Build history of the part. All positions in model axes, mm. A direction names the side the tool comes from. Round coordinates to 2 decimals unless told otherwise and drop trailing zeros. Write each loop counter-clockwise with the first axis right and the second up, starting at its lowest first coordinate (ties: lowest second). Pieces come first, ordered by that corner, then holes. Notation, with made-up numbers: (55, 9) -> (98, 9) arc R31 cw to (98, 44) -> close; hole circle Ø1 at (5, 22.25). An arc over 180 degrees is marked (long way). One line per question, with ' | ' between items.
from build123d import *

# Parameters (mm, degrees)
F0_W     = 63.5
F0_H     = 38.1
F1_DEPTH = 25.4
F3_DEPTH = 25.4


with BuildPart() as f1:
    # F0 (on Front) → F1 (new body)
    with BuildSketch(Plane.XZ):
        with Locations((-31.75, 19.05)):
            Rectangle(F0_W, F0_H)
    extrude(amount=F1_DEPTH)

    # F2 (on face) → F3 (cut)
    with BuildSketch(Plane.XZ.offset(25.4)):
        with BuildLine():
            ThreePointArc((-50.8, 38.1), (-44.931719, 24.918281), (-31.75, 19.05))
            ThreePointArc((-31.75, 19.05), (-18.530061, 24.880061), (-12.7, 38.1))
            Line((-12.7, 38.1), (-31.75, 38.1))
            Line((-31.75, 38.1), (-50.8, 38.1))
        make_face()
    extrude(amount=-F3_DEPTH, mode=Mode.SUBTRACT)


solid = f1.part
(1) 3-axis set-ups, long thin cutter, end or side, ignore diameter. For faces 1 (the cylindrical face through (-45.08, -12.88, 25.07)), 2 (the flat face through (-32, -13, 0)): which of +Z, -Z, +X, -X, +Y, -Y reach the whole face in a straight line?
Calculated:
face 1: +Z, +Y, -Y | face 2: -Z, +X, -X, +Y, -Y
(2) Slice it at C-C (x = -46.5). Write the cut outline in (y, z).
Calculated:
outline: (-25.4, 0) -> (0, 0) -> (0, 26.68) -> (-25.4, 26.68) -> close
(3) Slice it at D-D (z = 33). Write the cut outline in (x, y).
Calculated:
outline: (-63.5, -25.4) -> (-49.86, -25.4) -> (-49.86, 0) -> (-63.5, 0) -> close; (-13.6, -25.4) -> (0, -25.4) -> (0, 0) -> (-13.6, 0) -> close
(4) Wall check: line 1 (X direction, y = -2, z = 26); line 2 (X direction, y = -22.75, z = 31); line 3 (Z direction, x = -35.5, y = -11). Give the ranges that are in metal, low to high. Write a range as from..to.
Calculated:
line 1: -63.5..-45.94, -17.49..0 | line 2: -63.5..-49.1, -14.35..0 | line 3: 0..19.6
(5) Slice it at A-A (z = 26.5). Write the cut outline in (x, y).
Calculated:
outline: (-63.5, -25.4) -> (-46.35, -25.4) -> (-46.35, 0) -> (-63.5, 0) -> close; (-17.08, -25.4) -> (0, -25.4) -> (0, 0) -> (-17.08, 0) -> close
(6) Slice it at B-B (y = -13). Write the cut outline in (x, z), then the cut area to 3 significant figures.
Calculated:
outline: (-63.5, 0) -> (0, 0) -> (0, 38.1) -> (-12.7, 38.1) arc R19.98 cw to (-31.75, 19.05) arc R20.13 cw to (-50.8, 38.1) -> (-63.5, 38.1) -> close | area: 1,860 mm2
